Geometry: final body of the model. Coordinates: model frame, mm. A direction names the side the tool comes from. Give positions to 0.01 mm unless a question says otherwise; leave off trailing zeros. Write each loop counter-clockwise with the first axis right and the second up, starting at its lowest first coordinate (ties: lowest second). Pieces come first, ordered by that corner, then holes. Notation, with made-up numbers: M -4.75,24.5 L 11.25,24.5 A28 ccw 11.25,43.5 Z; hole C 9.5,34 d8. An arc over 180 degrees is marked long. Use one line per item in the form item = value. Start each with the question number.
Item 1: Section query C-C on x = -41. Return loops of the section in (y, z), then the cut area to 3 significant figures.
Item 2: Pull-direction query (X, two-part tool) for faces 4 (the cylindrical face through (-20.24, 4.93, 4.94)), 5 (the cylindrical face through (27.2, 4.93, -12.77)), 6 (the cylindrical face through (17.565, 4.93, -33.345)); classes: released by +X, released by -X, zero draft, split by the parting line, or undercut.
Item 3: Section query A-A on x = 2. Return loops of the section in (y, z), then the cut area to 3 significant figures.
Item 4: Access query for faces 1 (the cylindrical face through (6.9, 4.93, -0.53)), 2 (the cylindrical face through (-30.324, 4.93, -3.867)), 3 (the flat face through (-0.4, 4.9, 21.6)). Directions: +Z, -Z, +X, -X, +Y, -Y. A direction counts if a zero-diameter tool reaches every point of the face in a straight line with its end or side. Return the directions, or none.
Item 5: Contact query for flat-ended pins moving along their axis: P1, Ø3, axis at y = 5, z = 19, coming from the +X side; P2, Ø6, axis at y = 3, z = -27, coming from the -X side. Output: stop coordinate, or through.
Item 6: Section query D-D on x = -26.5. Return loops of the section in (y, z).
Item 7: Section query B-B on y = 7.5. Return loops of the section in (x, z) (1 decimal).
Item 8: Material intervals for line 1 along Z through (x, y) = (10.5, 6.75); line 2 along X through (y, z) = (3.75, 9.5); line 3 along X through (y, z) = (6, 14), sorted ascending. Write a range as from..to.
from build123d import *

# Parameters (mm, degrees)
SKETCH1_R           = 6.5
SKETCH1_R_2         = 8
BOSS_EXTRUDE1_DEPTH = 10


with BuildPart() as part:
    # Sketch1 → Boss-Extrude1 (new body)
    with BuildSketch(Plane(origin=(0, 0, 0), x_dir=(1, 0, 0), z_dir=(0, 1, 0))):
        with BuildLine():
            Line((34.360854191, -1.561869431), (30.455482575, 4.991720076))
            ThreePointArc((30.455482575, 4.991720076), (27.168828712, 12.889530967), (26.244815541, 21.393865753))
            ThreePointArc((26.244815541, 21.393865753), (17.347223993, 33.405750066), (3.646755092, 27.426648798))
            ThreePointArc((3.646755092, 27.426648798), (-1.375508537, 20.532192172), (-8.135127404, 15.329864146))
            Line((-8.135127404, 15.329864146), (-23.489726911, 6.674621202))
            ThreePointArc((-23.489726911, 6.674621202), (-30.425083941, 3.839275852), (-37.846730781, 2.810918636))
            ThreePointArc((-37.846730781, 2.810918636), (-48.587233234, -9.823261281), (-34.60716777, -18.741706478))
            ThreePointArc((-34.60716777, -18.741706478), (-27.816143316, -17.570430421), (-20.937015372, -17.979697402))
            Line((-20.937015372, -17.979697402), (20.632426372, -25.309509119))
            ThreePointArc((20.632426372, -25.309509119), (27.032722198, -27.191241227), (32.858920246, -30.440874852))
            ThreePointArc((32.858920246, -30.440874852), (48.469635541, -27.492571895), (44.854019442, -12.022787068))
            ThreePointArc((44.854019442, -12.022787068), (38.951456853, -7.450330386), (34.360854191, -1.561869431))
        make_face()
        with Locations(Location((-37.709427644, -8.188224414, 0), (0, 0, 270))):
            Circle(SKETCH1_R, mode=Mode.SUBTRACT)
        with Locations(Location((14.252094878, 21.811778539, 0), (0, 0, 270))):
            Circle(SKETCH1_R_2, mode=Mode.SUBTRACT)
        with Locations(Location((39.252097338, -21.489490229, 0), (0, 0, 270))):
            Circle(SKETCH1_R, mode=Mode.SUBTRACT)
        with BuildLine():
            Line((20.312704962, -21.992225916), (-19.891412958, -15.327696302))
            ThreePointArc((-19.891412958, -15.327696302), (-23.883928025, -11.759574594), (-22.359792068, -6.626478193))
            ThreePointArc((-22.359792068, -6.626478193), (-20.208737863, -4.917702185), (-17.910389919, -3.41286121))
            Line((-17.910389919, -3.41286121), (-16.434238636, -2.540199474))
            ThreePointArc((-16.434238636, -2.540199474), (7.233462597, 0.434776311), (25.58991918, -14.798446076))
            ThreePointArc((25.58991918, -14.798446076), (25.161933747, -20.017004215), (20.312704962, -21.992225916))
        make_face(mode=Mode.SUBTRACT)
    extrude(amount=BOSS_EXTRUDE1_DEPTH)


solid = part.part
Answer sheet:
q1.outline = M 0,-2.31 L 10,-2.31 L 10,2.58 L 0,2.58 Z; M 0,13.79 L 10,13.79 L 10,18.68 L 0,18.68 Z
q1.area = 97.8 mm2
q2.face_4 = undercut
q2.face_5 = released by +X
q2.face_6 = split by the parting line
q3.outline = M 0,-24.68 L 10,-24.68 L 10,-1.47 L 0,-1.47 Z; M 0,18.96 L 10,18.96 L 10,22.02 L 0,22.02 Z
q3.area = 263 mm2
q4.face_1 = +Y, -Y
q4.face_2 = -Z, -X, +Y, -Y
q4.face_3 = +Z, +Y, -Y
q5.P1 = 50.21
q5.P2 = 1.53
q6.outline = M 0,-5.19 L 10,-5.19 L 10,17.53 L 0,17.53 Z
q7.outline = M -37.8,-2.8 A30 cw -23.5,-6.7 L -8.1,-15.3 A30 cw 3.6,-27.4 A12 ccw 26.2,-21.4 A30 cw 30.5,-5 L 34.4,1.6 A30 cw 44.9,12 A11 ccw long 32.9,30.4 A30 cw 20.6,25.3 L -20.9,18 A30 cw -34.6,18.7 A11 ccw long Z; hole C -37.7,8.2 d13; hole M -22.4,6.6 A30 ccw -17.9,3.4 L -16.4,2.5 A30 ccw 25.6,14.8 A5 ccw 20.3,22 L -19.9,15.3 A5 ccw Z; hole C 14.3,-21.8 d16; hole C 39.3,21.5 d13
q8.line_1 = -33.21..-28.88, -14.75..0.73, 20.37..23.52
q8.line_2 = -48.63..-44.08, -31.34..-23.99, 22.16..41.23
q8.line_3 = -47.05..-40.62, -34.8..-22.54, 25.17..47.31
